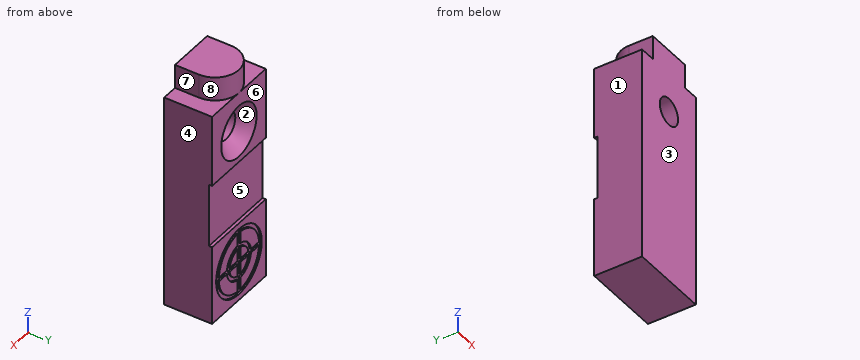
from build123d import *

# Parameters (mm, degrees)
SKETCH_1_W                = 10
SKETCH_1_H                = 27
SKETCH_1_R                = 1.5
EXTRUDE_1_DEPTH           = 6
SKETCH_2_R                = 4.25
SKETCH_2_R_2              = 3.75
SKETCH_2_R_3              = 2.25
SKETCH_2_R_4              = 1.75
SKETCH_2_W                = 8
SKETCH_2_H                = 0.5
SKETCH_2_W_2              = 0.5
SKETCH_2_H_2              = 8
CUT_EXTRUDE_1_DEPTH       = 0.2
SKETCH_3_W                = 10
SKETCH_3_H                = 8
CUT_EXTRUDE_1_2_DEPTH     = 0.4
HOLE_WIZARD_1_D           = 3.4
HOLE_WIZARD_1_DEPTH       = 22.25
HOLE_WIZARD_1_CSINK_D     = 6.6
HOLE_WIZARD_1_CSINK_ANGLE = 90
HOLE_WIZARD_1_TIP         = 1.021463052
EXTRUDE_2_DEPTH           = 3


with BuildPart() as part:
    # 草图1 → 凸台-拉伸1 (new body)
    with BuildSketch(Plane(origin=(0, 0, 0), x_dir=(1, 0, 0), z_dir=(0, 1, 0))):
        with Locations((5, 13.5)):
            Rectangle(SKETCH_1_W, SKETCH_1_H)
        with Locations(Location((5, 5, 0), (0, 0, 270))):
            Circle(SKETCH_1_R, mode=Mode.SUBTRACT)
    extrude(amount=EXTRUDE_1_DEPTH)

    # 草图2 → Cut-Extrude 1 (cut)
    # profile 1 of 4: a face of its own
    with BuildSketch(Plane(origin=(0, 6, 0), x_dir=(1, 0, 0), z_dir=(0, 1, 0))):
        with Locations((5, 22)):
            Circle(SKETCH_2_R)
        with Locations((5, 22)):
            Circle(SKETCH_2_R_2, mode=Mode.SUBTRACT)
    # profile 2 of 4: a face of its own
    with BuildSketch(Plane(origin=(0, 6, 0), x_dir=(1, 0, 0), z_dir=(0, 1, 0))):
        with Locations((5, 22)):
            Circle(SKETCH_2_R_3)
        with Locations((5, 22)):
            Circle(SKETCH_2_R_4, mode=Mode.SUBTRACT)
    # profile 3 of 4: a face of its own
    with BuildSketch(Plane(origin=(0, 6, 0), x_dir=(1, 0, 0), z_dir=(0, 1, 0))):
        with Locations((5, 22)):
            Rectangle(SKETCH_2_W, SKETCH_2_H)
    # profile 4 of 4: a face of its own
    with BuildSketch(Plane(origin=(0, 6, 0), x_dir=(1, 0, 0), z_dir=(0, 1, 0))):
        with Locations((5, 22)):
            Rectangle(SKETCH_2_W_2, SKETCH_2_H_2)
    extrude(amount=-CUT_EXTRUDE_1_DEPTH, mode=Mode.SUBTRACT)

    # 草图3 → Cut-Extrude 1 2 (cut)
    with BuildSketch(Plane(origin=(0, 6, 0), x_dir=(1, 0, 0), z_dir=(0, 1, 0))):
        with Locations((5, 13)):
            Rectangle(SKETCH_3_W, SKETCH_3_H)
    extrude(amount=-CUT_EXTRUDE_1_2_DEPTH, mode=Mode.SUBTRACT)

    # 打孔尺寸(%根据十字)槽半沉头木螺钉的类型1
    with Locations(Plane(origin=(0, 6, 0), x_dir=(1, 0, 0), z_dir=(0, 1, 0))):
        with Locations((5, 5)):
            CounterSinkHole(HOLE_WIZARD_1_D / 2, HOLE_WIZARD_1_CSINK_D / 2, depth=HOLE_WIZARD_1_DEPTH, counter_sink_angle=HOLE_WIZARD_1_CSINK_ANGLE)
            with Locations((0, 0, -(HOLE_WIZARD_1_DEPTH + HOLE_WIZARD_1_TIP / 2))):  # 118° drill point
                Cone(0, HOLE_WIZARD_1_D / 2, HOLE_WIZARD_1_TIP, mode=Mode.SUBTRACT)

    # 草图6 → 凸台-拉伸2 (add)
    with BuildSketch(Plane.XY):
        with BuildLine():
            Line((2, 3), (2, 0))
            Line((2, 0), (8, 0))
            Line((8, 0), (8, 3))
            ThreePointArc((8, 3), (5, 6), (2, 3))
        make_face()
    extrude(amount=EXTRUDE_2_DEPTH)


solid = part.part
Verification items for the finished model (mm, model axes). Face numbers are marked on the shaded views. A direction names the side the tool comes from. Give positions to 0.01 mm unless a question says otherwise; leave off trailing zeros. Loops run counter-clockwise (first coordinate to the right, second up) from the corner with the lowest first, then second, coordinate; pieces in that order, holes last. Notation, with made-up numbers: (-22.5, 53.5) - (-17.5, 53.5) arc R23 cw to (-17.5, 61.5) - close; hole circle Ø10 at (48.5, 67). An arc over 180 degrees is marked (long way). Write each question's results on one line, items separated by ' | '.
1) Material ranges on L1, parallel to Z at x = 5, y = 5.95; L2, parallel to X at y = 3.3, z = -5; L3, parallel to X at y = 5.9, z = -22, recorded low to high. Write a range as from..to.
Solution:
L1: -27..-26.25, -17.75..-17, -9..-8.25, -1.75..3 | L2: 0..3.3, 6.7..10 | L3: 0..0.75, 9.25..10
2) Depth check by flat-ended pin: P1, Ø2.5, axis at x = 5, z = -11, coming from the +Y side; P2, Ø3, axis at x = 5, z = -5, coming from the +Y side. Enter the tip coordinate at first touch or a pass-through.
Solution:
P1: y = 5.6 | P2: through
3) Sectioned sample at B-B on z = -11.5. Record the boundary of the cut face in (x, y).
Solution:
outline: (0, 0) - (10, 0) - (10, 5.6) - (0, 5.6) - close
4) Tool access check on the marked faces 4, 5, 6, 7 and 8. Record the directions out of +Z, -Z, +X, -X, +Y, -Y that give a thin tool (end or side, any length) a straight path to the whole face; none if there is none.
Solution:
face 4: +Z, -Z, +X, +Y, -Y | face 5: +X, -X, +Y | face 6: +Z, -Z, +X, -X, +Y | face 7: +Z, +X, +Y, -Y | face 8: +Z, +Y
5) Sectioned sample at A-A on z = 1. Record the boundary of the cut face in (x, y).
Solution:
outline: (2, 0) - (8, 0) - (8, 3) arc R3 ccw to (2, 3) - close
6) Mould release check, pull along X, two halves, no side actions. Record for the marked faces 1, 2 and 3: pulls with the +X half, pulls with the -X half, needs draft (parallel to the pull), parting line crosses it, or undercut.
Solution:
face 1: pulls with the -X half | face 2: undercut | face 3: needs draft
